Could you check a few things on this model? Use its own coordinates, in mm. Give positions to 0.01 mm unless a question says otherwise; leave off trailing zeros. Loops run counter-clockwise (first coordinate to the right, second up) from the corner with the lowest first, then second, coordinate; pieces in that order, holes last. Notation, with made-up numbers: (-34, 13) -> (16, 13) arc R17 cw to (16, 21) -> close; hole circle Ø2 at (55.5, 4). An arc over 180 degrees is marked (long way). Put each result on its own line as item: value.
```python
from build123d import *

# Parameters (mm, degrees)
ESQUISSE1_R             = 1.5
BOSS_EXTRU_2_DEPTH      = 5
ESQUISSE2_W             = 5
ESQUISSE2_H             = 140
BOSS_EXTRU_3_DEPTH      = 5
ESQUISSE3_W             = 5
ESQUISSE3_H             = 140
BOSS_EXTRU_4_DEPTH      = 5
ESQUISSE4_W             = 3.5
ESQUISSE4_H             = 3
ESQUISSE4_W_2           = 3
ESQUISSE4_H_2           = 1
ENL_V_MAT_EXTRU_1_DEPTH = 10


with BuildPart() as part:
    # Esquisse1 → Boss.-Extru.2 (new body)
    with BuildSketch(Plane.XY):
        with BuildLine():
            Line((-160.623123651, 88.85383225), (-160.623123651, -51.14616775))
            Line((-160.623123651, -51.14616775), (-105.623123651, -51.14616775))
            Line((-105.623123651, -51.14616775), (-105.623123651, -56.14616775))
            Line((-105.623123651, -56.14616775), (-92.281436046, -56.14616775))
            ThreePointArc((-92.281436046, -56.14616775), (-90.623123651, -56.64616775), (-88.964811256, -56.14616775))
            Line((-88.964811256, -56.14616775), (-75.623123651, -56.14616775))
            Line((-75.623123651, -56.14616775), (-75.623123651, -51.14616775))
            Line((-75.623123651, -51.14616775), (44.376876349, -51.14616775))
            Line((44.376876349, -51.14616775), (44.376876349, -56.14616775))
            Line((44.376876349, -56.14616775), (57.718563954, -56.14616775))
            ThreePointArc((57.718563954, -56.14616775), (59.376876349, -56.64616775), (61.035188744, -56.14616775))
            Line((61.035188744, -56.14616775), (74.376876349, -56.14616775))
            Line((74.376876349, -56.14616775), (74.376876349, -51.14616775))
            Line((74.376876349, -51.14616775), (129.376876349, -51.14616775))
            Line((129.376876349, -51.14616775), (129.376876349, 88.85383225))
            Line((129.376876349, 88.85383225), (74.376876349, 88.85383225))
            Line((74.376876349, 88.85383225), (74.376876349, 93.85383225))
            Line((74.376876349, 93.85383225), (61.035188744, 93.85383225))
            ThreePointArc((61.035188744, 93.85383225), (59.376876349, 94.35383225), (57.718563954, 93.85383225))
            Line((57.718563954, 93.85383225), (44.376876349, 93.85383225))
            Line((44.376876349, 93.85383225), (44.376876349, 88.85383225))
            Line((44.376876349, 88.85383225), (-75.623123651, 88.85383225))
            Line((-75.623123651, 88.85383225), (-75.623123651, 93.85383225))
            Line((-75.623123651, 93.85383225), (-88.964811256, 93.85383225))
            ThreePointArc((-88.964811256, 93.85383225), (-90.623123651, 94.35383225), (-92.281436046, 93.85383225))
            Line((-92.281436046, 93.85383225), (-105.623123651, 93.85383225))
            Line((-105.623123651, 93.85383225), (-105.623123651, 88.85383225))
            Line((-105.623123651, 88.85383225), (-160.623123651, 88.85383225))
        make_face()
        with Locations((-90.623123651, -53.64616775)):
            Circle(ESQUISSE1_R, mode=Mode.SUBTRACT)
        with Locations((59.376876349, -53.64616775)):
            Circle(ESQUISSE1_R, mode=Mode.SUBTRACT)
        with Locations((-90.623123651, 91.35383225)):
            Circle(ESQUISSE1_R, mode=Mode.SUBTRACT)
        with Locations((59.376876349, 91.35383225)):
            Circle(ESQUISSE1_R, mode=Mode.SUBTRACT)
    extrude(amount=BOSS_EXTRU_2_DEPTH)

    # Esquisse2 → Boss.-Extru.3 (add)
    with BuildSketch(Plane.ZY.offset(160.623123651)):
        with Locations((2.5, 18.85383225)):
            Rectangle(ESQUISSE2_W, ESQUISSE2_H)
    extrude(amount=BOSS_EXTRU_3_DEPTH)

    # Esquisse3 → Boss.-Extru.4 (add)
    with BuildSketch(Plane(origin=(129.376876349, 0, 0), x_dir=(0, 0, -1), z_dir=(1, 0, 0))):
        with Locations((-2.5, 18.85383225)):
            Rectangle(ESQUISSE3_W, ESQUISSE3_H)
    extrude(amount=BOSS_EXTRU_4_DEPTH)

    # Esquisse4 → Enlèv. mat.-Extru.1 (cut)
    with BuildSketch(Plane.XY.offset(5)):
        Polygon((-165.623123651, 33.85383225), (-165.623123651, 3.85383225), (-160.623123651, 3.85383225), (-160.623123651, 17.35383225), (-160.623123651, 20.35383225), (-160.623123651, 33.85383225), align=None)
        with Locations((-158.873123651, 18.85383225)):
            Rectangle(ESQUISSE4_W, ESQUISSE4_H)
        with Locations((-155.623123651, 18.85383225)):
            Rectangle(ESQUISSE4_W_2, ESQUISSE4_H)
        with Locations((-155.623123651, 20.85383225)):
            Rectangle(ESQUISSE4_W_2, ESQUISSE4_H_2)
        with Locations((-155.623123651, 16.85383225)):
            Rectangle(ESQUISSE4_W_2, ESQUISSE4_H_2)
        with Locations((-152.373123651, 18.85383225)):
            Rectangle(ESQUISSE4_W, ESQUISSE4_H)
        Polygon((129.376876349, 20.35383225), (129.376876349, 17.35383225), (129.376876349, 3.85383225), (134.376876349, 3.85383225), (134.376876349, 33.85383225), (129.376876349, 33.85383225), align=None)
        with Locations((127.626876349, 18.85383225)):
            Rectangle(ESQUISSE4_W, ESQUISSE4_H)
        with Locations((124.376876349, 18.85383225)):
            Rectangle(ESQUISSE4_W_2, ESQUISSE4_H)
        with Locations((124.376876349, 20.85383225)):
            Rectangle(ESQUISSE4_W_2, ESQUISSE4_H_2)
        with Locations((124.376876349, 16.85383225)):
            Rectangle(ESQUISSE4_W_2, ESQUISSE4_H_2)
        with Locations((121.126876349, 18.85383225)):
            Rectangle(ESQUISSE4_W, ESQUISSE4_H)
    extrude(amount=-ENL_V_MAT_EXTRU_1_DEPTH, mode=Mode.SUBTRACT)


solid = part.part
```
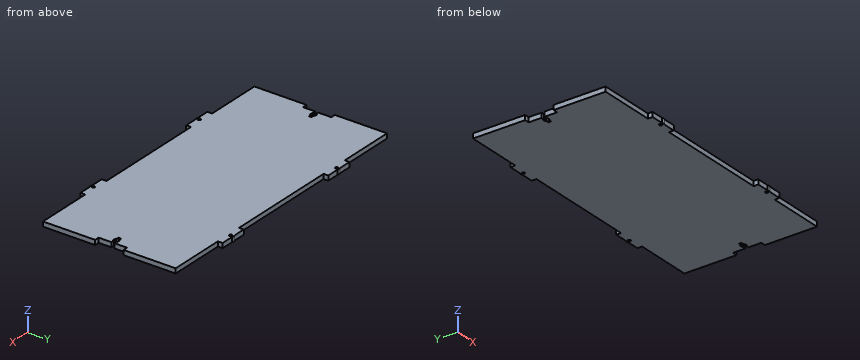
1. I need wall thicknesses on line 1 (Y direction, x = -45, z = 1.7); line 2 (X direction, y = 24, z = 3.15); line 3 (Y direction, x = 62, z = 4.6). Which ranges of each line are inside material? Lowest first, please.
Recorded:
line 1: y = -51.15 to 88.85
line 2: x = -160.62 to 129.38
line 3: y = -56.15 to 93.85
2. If we section it at B-B (x = -58.5): List the corners of the cut face in (y, z) for me.
Recorded:
outline: (-51.15, 0) -> (88.85, 0) -> (88.85, 5) -> (-51.15, 5) -> close
3. If we section it at C-C (z = 1.65): Count the separate pieces of the cut face and the enclosed holes in it, then the cut area to 3 significant figures.
Recorded:
separate pieces: 1
enclosed holes: 4
area: 42,200 mm^2
4. If we section it at A-A (y = 28): List the corners of the cut face in (x, z) for me.
Recorded:
outline: (-160.62, 0) -> (129.38, 0) -> (129.38, 5) -> (-160.62, 5) -> close
5. I'm going to push flat-ended pins straight in: pin 1 (1.5 mm diameter, centred on x = 64.5, z = 2, fed in from +Y); pin 2 (2.5 mm diameter, centred on x = -142.5, z = 3.5, fed in from +Y); pin 3 (2.5 mm diameter, centred on x = -4, z = 3.5, fed in from -Y). Where does each tip first touch, or does it pass through?
Recorded:
pin 1: stops at y = 93.85
pin 2: stops at y = 88.85
pin 3: stops at y = -51.15
